```python
from build123d import *

# Parameters (mm, degrees)
ESQUISSE1_W                  = 35
ESQUISSE1_H                  = 35
BOSS_EXTRU_1_DEPTH           = 11
ESQUISSE2_W                  = 16
ESQUISSE2_H                  = 10
ENL_V_MAT_EXTRU_1_DEPTH      = 34.667491739
ESQUISSE3_R                  = 2
ENL_V_MAT_EXTRU_2_DEPTH      = 50
ENL_V_MAT_EXTRU_3_DEPTH      = 52.500000152
ENL_V_MAT_EXTRU_3_DEPTH_BACK = 40


with BuildPart() as part:
    # Esquisse1 → Boss.-Extru.1 (new body)
    with BuildSketch(Plane.XY):
        with BuildLine():
            Line((17.5, -22.5), (-17.5, -22.5))
            ThreePointArc((-17.5, -22.5), (-21.035533906, -21.035533906), (-22.5, -17.5))
            Line((-22.5, -17.5), (-22.5, 17.5))
            ThreePointArc((-22.5, 17.5), (-21.035533906, 21.035533906), (-17.5, 22.5))
            Line((-17.5, 22.5), (17.5, 22.5))
            ThreePointArc((17.5, 22.5), (21.035533906, 21.035533906), (22.5, 17.5))
            Line((22.5, 17.5), (22.5, -17.5))
            ThreePointArc((22.5, -17.5), (21.035533906, -21.035533906), (17.5, -22.5))
        make_face()
        Rectangle(ESQUISSE1_W, ESQUISSE1_H, mode=Mode.SUBTRACT)
    extrude(amount=BOSS_EXTRU_1_DEPTH)

    # Esquisse2 → Enlèv. mat.-Extru.1 (cut, through all)
    with BuildSketch(Plane.XY.offset(11)):
        with Locations((0, 20.5)):
            Rectangle(ESQUISSE2_W, ESQUISSE2_H)
    extrude(amount=-ENL_V_MAT_EXTRU_1_DEPTH, mode=Mode.SUBTRACT)

    # Esquisse3 → Enlèv. mat.-Extru.2 (cut, symmetric)
    with BuildSketch(Plane(origin=(-8, 0, 0), x_dir=(0, 0, -1), z_dir=(1, 0, 0))):
        with Locations(Location((-5.5, 20, 0), (0, 0, 90))):
            Circle(ESQUISSE3_R)
    extrude(amount=ENL_V_MAT_EXTRU_2_DEPTH, both=True, mode=Mode.SUBTRACT)

    # Esquisse4 → Enlèv. mat.-Extru.3 (cut, two sides: drawn at the far end of the back side and taken through both)
    with BuildSketch(Plane.XZ.offset(22.5).offset(-ENL_V_MAT_EXTRU_3_DEPTH_BACK)):
        with BuildLine():
            Line((10.5, 11), (0, 11))
            Line((0, 11), (0, 2))
            Line((0, 2), (8.5, 2))
            ThreePointArc((8.5, 2), (9.914213562, 2.585786438), (10.5, 4))
            Line((10.5, 4), (10.5, 11))
        make_face()
        with BuildLine():
            Line((0, 11), (-10.5, 11))
            Line((-10.5, 11), (-10.5, 4))
            ThreePointArc((-10.5, 4), (-9.914213562, 2.585786438), (-8.5, 2))
            Line((-8.5, 2), (0, 2))
            Line((0, 2), (0, 11))
        make_face()
    extrude(amount=ENL_V_MAT_EXTRU_3_DEPTH + ENL_V_MAT_EXTRU_3_DEPTH_BACK, mode=Mode.SUBTRACT)


solid = part.part
```
The listing builds one solid part. Answer for the finished solid, in the listing's coordinates (mm). A direction names the side the tool comes from. Round coordinates to 2 decimals unless told otherwise and drop trailing zeros. Loops run counter-clockwise (first coordinate to the right, second up) from the corner with the lowest first, then second, coordinate; pieces in that order, holes last.
Q1. Find the intervals of material crossed by line 1 (Y direction, x = -12, z = 5.5); line 2 (Y direction, x = 13, z = 8.5), in increasing order.
Q2. Section C-C, the plane z = 1 is taken. Determine the outline of the cut face in (x, y), then the cut area to 3 significant figures.
Q3. Given pin 1 Ø1.5 at (y, z) = (21, 4) entering from +X; pin 2 Ø5.5 at (y, z) = (21, 3) entering from -X; pin 3 Ø3.5 at (y, z) = (20, 5.5) entering from +X; pin 4 Ø5.5 at (x, y) = (-1, -21) entering from +Z, each flat-ended and moving along its own axis, determine where each tip first touches the part or whether it passes through.
Q4. Section A-A, the plane y = -8 is taken. Determine the outline of the cut face in (x, z).
Q5. For a pull along Y with two mould halves and no side action, classify faces 6 (the face through (-13, 17.5, 5)), 7 (the face through (0.2, -22.5, 1.8)), 8 (the face through (-17.5, 0, 5)), 9 (the face through (22.5, 0, 5)) as released by +Y, released by -Y, zero draft, split by the parting line, or undercut.
Q6. Which of the six approach directions +Z, -Z, +X, -X, +Y, -Y give full straight-line access (tool end or side, diameter ignored) to faces 1 (the face through (8, 18, 7)), 2 (the face through (10.5, -20, 7)), 3 (the face through (19.563, 22.054, 4.201)), 4 (the face through (21.07, -21, 5.42)), 5 (the face through (13, 17.5, 5))?
Q7. Section B-B, the plane z = 8.25 is taken. Determine the outline of the cut face in (x, y).
Q8. Section D-D, the plane x = -18.5 is taken. Determine the outline of the cut face in (y, z).
Completed:
1. line 1: y = -22.5 to -17.5, 17.5 to 18, 22 to 22.5
1. line 2: y = -22.5 to -17.5, 17.5 to 22.5
2. outline: (-22.5, -17.5) arc R5 ccw to (-17.5, -22.5) - (17.5, -22.5) arc R5 ccw to (22.5, -17.5) - (22.5, 17.5) arc R5 ccw to (17.5, 22.5) - (8, 22.5) - (8, 17.5) - (17.5, 17.5) - (17.5, -17.5) - (-17.5, -17.5) - (-17.5, 17.5) - (-8, 17.5) - (-8, 22.5) - (-17.5, 22.5) arc R5 ccw to (-22.5, 17.5) - close
2. area: 699 mm2
3. pin 1: stops at x = 21.57
3. pin 2: stops at x = -22.44
3. pin 3: passes through
3. pin 4: stops at z = 2
4. outline: (-22.5, 0) - (-17.5, 0) - (-17.5, 11) - (-22.5, 11) - close; (17.5, 0) - (22.5, 0) - (22.5, 11) - (17.5, 11) - close
5. face 6: undercut
5. face 7: released by -Y
5. face 8: undercut
5. face 9: zero draft
6. face 1: +Z, -Z, +Y
6. face 2: +Z, -Y
6. face 3: +Z, -Z, +X, +Y
6. face 4: +Z, -Z, +X, -Y
6. face 5: +Z, -Z
7. outline: (-22.5, -17.5) arc R5 ccw to (-17.5, -22.5) - (-10.5, -22.5) - (-10.5, -17.5) - (-17.5, -17.5) - (-17.5, 17.5) - (-8, 17.5) - (-8, 22.5) - (-17.5, 22.5) arc R5 ccw to (-22.5, 17.5) - close; (8, 17.5) - (17.5, 17.5) - (17.5, -17.5) - (10.5, -17.5) - (10.5, -22.5) - (17.5, -22.5) arc R5 ccw to (22.5, -17.5) - (22.5, 17.5) arc R5 ccw to (17.5, 22.5) - (8, 22.5) - close
8. outline: (-22.4, 0) - (22.4, 0) - (22.4, 11) - (-22.4, 11) - close; hole circle Ø4 at (20, 5.5)
